from build123d import *

# Parameters (mm, degrees)
SKETCH_1_W                  = 413.2
SKETCH_1_H                  = 588.12
EXTRUDE_1_DEPTH             = 1.2
CUT_EXTRUDE_1_DEPTH         = 360.383198828
CUT_EXTRUDE_1_DEPTH_BACK    = 360.383198828
EXTRUDE_3_DEPTH             = 413.2
CUT_EXTRUDE_2_REACH         = 407.539
SKETCH_5_W                  = 413.2
SKETCH_5_H                  = 1
HOLE_WIZARD_M5_1_AT_2_COUNT = 2
HOLE_WIZARD_M5_1_AT_2_PITCH = 250
HOLE_WIZARD_M5_1_AT_3_COUNT = 2
HOLE_WIZARD_M5_1_AT_3_PITCH = 436.48692993
HOLE_WIZARD_M5_1_AT_4_COUNT = 2
HOLE_WIZARD_M5_1_AT_4_PITCH = 357.8
CUT_EXTRUDE_3_REACH         = 553.095
SKETCH_10_W                 = 80
SKETCH_10_H                 = 49
CUT_EXTRUDE_4_REACH         = 665.873
SKETCH_11_W                 = 20
SKETCH_11_H                 = 60
CUT_EXTRUDE_5_DEPTH         = 20


with BuildPart() as part:
    # 스케치1 → 보스-돌출1 (new body)
    with BuildSketch(Plane(origin=(0, 0, 0), x_dir=(1, 0, 0), z_dir=(0, 1, 0))):
        Rectangle(SKETCH_1_W, SKETCH_1_H)
    extrude(amount=EXTRUDE_1_DEPTH)

    # 스케치2 → 컷-돌출1 (cut, two sides: drawn at the far end of the back side and taken through both)
    with BuildSketch(Plane(origin=(0, 0, 0), x_dir=(0, 0, -1), z_dir=(1, 0, 0)).offset(-CUT_EXTRUDE_1_DEPTH_BACK)):
        Polygon((-293.957235481, 0), (-293.673125179, 1.2), (-294.06, 1.2), (-294.06, 0), align=None)
    extrude(amount=CUT_EXTRUDE_1_DEPTH + CUT_EXTRUDE_1_DEPTH_BACK, mode=Mode.SUBTRACT)

    # 스케치4 → 보스-돌출3 (add)
    with BuildSketch(Plane(origin=(206.6, 0, 0), x_dir=(0, 0, -1), z_dir=(1, 0, 0))):
        with BuildLine():
            Line((-293.957235481, 0), (-314.720041398, -87.696105733))
            ThreePointArc((-314.720041398, -87.696105733), (-312.832491208, -96.20326758), (-304.989056289, -100))
            Line((-304.989056289, -100), (-195.633093997, -100))
            Line((-195.633093997, -100), (-195.633093997, -149))
            Line((-195.633093997, -149), (-194.433093997, -149))
            Line((-194.433093997, -149), (-194.433093997, -98.8))
            Line((-194.433093997, -98.8), (-304.989056289, -98.8))
            ThreePointArc((-304.989056289, -98.8), (-311.891279018, -95.45887547), (-313.552323185, -87.972573045))
            Line((-313.552323185, -87.972573045), (-292.789517268, -0.276467312))
            Line((-292.789517268, -0.276467312), (-292.724061259, 0))
            Line((-292.724061259, 0), (-293.957235481, 0))
        make_face()
    extrude(amount=-EXTRUDE_3_DEPTH)

    # 스케치5 → 컷-돌출2 (cut, up to next)
    with BuildSketch(Plane(origin=(0, 1.2, 0), x_dir=(1, 0, 0), z_dir=(0, 1, 0)), mode=Mode.PRIVATE) as cut_extrude_2_sk1:
        with Locations((0, 293.56)):
            Rectangle(SKETCH_5_W, SKETCH_5_H)
    cut_extrude_2_tool1 = extrude(cut_extrude_2_sk1.sketch, amount=-CUT_EXTRUDE_2_REACH, mode=Mode.PRIVATE) & part.part
    add(cut_extrude_2_tool1.solids().sort_by_distance((0, 1.2, -293.56))[0], mode=Mode.SUBTRACT)

    # 스케치8 → M5 접시 머리 나사용 카운터싱크1 (revolve, cut)
    with BuildSketch(Plane(origin=(-125, 1.2, -213.06), x_dir=(0, 0, 1), z_dir=(1, 0, 0))):
        Polygon((0, 0), (0, 1.2), (2.75, 1.2), (2.75, 2.75), (5.2, 0.3), (5.2, 0), align=None)
    hole_wizard_m5_1 = revolve(axis=Axis((-125, 7.55, -213.06), (0, -1, 0)), mode=Mode.SUBTRACT)

    # M5 접시 머리 나사용 카운터싱크1 at 2: M5 접시 머리 나사용 카운터싱크1 ×2
    with Locations(*[(i * HOLE_WIZARD_M5_1_AT_2_PITCH, 0, 0) for i in range(1, HOLE_WIZARD_M5_1_AT_2_COUNT)]):
        add(hole_wizard_m5_1, mode=Mode.SUBTRACT)

    # M5 접시 머리 나사용 카운터싱크1 at 3: M5 접시 머리 나사용 카운터싱크1 ×2
    with Locations(*[Vector(0.5727548360724275, 0, 0.8197267213868575) * (i * HOLE_WIZARD_M5_1_AT_3_PITCH) for i in range(1, HOLE_WIZARD_M5_1_AT_3_COUNT)]):
        add(hole_wizard_m5_1, mode=Mode.SUBTRACT)

    # M5 접시 머리 나사용 카운터싱크1 at 4: M5 접시 머리 나사용 카운터싱크1 ×2
    with Locations(*[(0, 0, i * HOLE_WIZARD_M5_1_AT_4_PITCH) for i in range(1, HOLE_WIZARD_M5_1_AT_4_COUNT)]):
        add(hole_wizard_m5_1, mode=Mode.SUBTRACT)

    # 스케치10 → 컷-돌출3 (cut, up to next)
    with BuildSketch(Plane.XY.offset(195.633093997), mode=Mode.PRIVATE) as cut_extrude_3_sk1:
        with Locations((0, -124.5)):
            Rectangle(SKETCH_10_W, SKETCH_10_H)
    cut_extrude_3_tool1 = extrude(cut_extrude_3_sk1.sketch, amount=-CUT_EXTRUDE_3_REACH, mode=Mode.PRIVATE) & part.part
    add(cut_extrude_3_tool1.solids().sort_by_distance((0, -124.5, 195.633094))[0], mode=Mode.SUBTRACT)

    # 컷-돌출4: up to this plane
    cut_extrude_4_end = Plane(origin=(-206.6, -0.276467312, 292.789517268), z_dir=(0, -0.2303894266765572, -0.9730985109821345))
    # 스케치11 → 컷-돌출4 (cut, up to the surface)
    with BuildSketch(Plane.XY.offset(320), mode=Mode.PRIVATE) as cut_extrude_4_sk1:
        with Locations((-136.6, -40)):
            Rectangle(SKETCH_11_W, SKETCH_11_H)
    cut_extrude_4_tool1 = split(extrude(cut_extrude_4_sk1.sketch, amount=-CUT_EXTRUDE_4_REACH, mode=Mode.PRIVATE), bisect_by=cut_extrude_4_end, keep=Keep.BOTH, mode=Mode.PRIVATE)
    add(cut_extrude_4_tool1.solids().sort_by_distance((-136.6, -40, 320))[0], mode=Mode.SUBTRACT)
    # 스케치11 → 컷-돌출4 (cut, up to the surface)
    with BuildSketch(Plane.XY.offset(320), mode=Mode.PRIVATE) as cut_extrude_4_sk2:
        with Locations((136.6, -40)):
            Rectangle(SKETCH_11_W, SKETCH_11_H)
    cut_extrude_4_tool2 = split(extrude(cut_extrude_4_sk2.sketch, amount=-CUT_EXTRUDE_4_REACH, mode=Mode.PRIVATE), bisect_by=cut_extrude_4_end, keep=Keep.BOTH, mode=Mode.PRIVATE)
    add(cut_extrude_4_tool2.solids().sort_by_distance((136.6, -40, 320))[0], mode=Mode.SUBTRACT)

    # 스케치12 → 컷-돌출5 (cut)
    with BuildSketch(Plane(origin=(-146.6, 0, 0), x_dir=(0, 0, -1), z_dir=(1, 0, 0))):
        Polygon((-295.09164711, -10), (-296.259365323, -9.723532688), (-296.324821333, -10), (-310.530336442, -70), (-309.316935211, -70.083515414), (-309.297162219, -70), align=None)
    cut_extrude_5 = extrude(amount=CUT_EXTRUDE_5_DEPTH, mode=Mode.SUBTRACT)

    # 대칭 복사2: 컷-돌출5 across plane
    add(cut_extrude_5.mirror(Plane(origin=(0, 0, 0), x_dir=(0, 0, 1), z_dir=(1, 0, 0))), mode=Mode.SUBTRACT)


solid = part.part
Part model, mm, in its own coordinate system. Give positions to 0.01 mm unless a question says otherwise; leave off trailing zeros. Loops run counter-clockwise (first coordinate to the right, second up) from the corner with the lowest first, then second, coordinate; pieces in that order, holes last. Notation, with made-up numbers: (50.5, 33.25) -> (75.5, 33.25) arc R31 ccw to (75.5, 71.25) -> close; hole circle Ø5 at (79, -18). An arc over 180 degrees is marked (long way). Write each question's results on one line, items separated by ' | '. Start each with the question number.
Q1. Band-saw the part on B-B on x = 47.5. List the corners of the cut face in (y, z).
Q2. Pin check, flat tips, straight feed: P1, Ø24.5, axis at x = 96, y = -131.5, coming from the +Z side; P2, Ø2, axis at x = -38.5, y = -127, coming from the -Z side; P3, Ø12, axis at x = 125, z = 144.74, coming from the -Y side; P4, Ø4, axis at x = -97, y = -59.5, coming from the -Z side. Stop position of each tip, or through.
Q3. Wall check: L1, parallel to X at y = 1, z = 144; L2, parallel to Z at x = 125, y = 1; L3, parallel to X at y = 1.05, z = 144.74. Give the ranges that are in metal, low to high.
Q4. Band-saw the part on D-D on z = 77.5. List the corners of the cut face in (x, y).
Q5. Band-saw the part on A-A on y = -126. List the corners of the cut face in (x, z), plus the area to 3 significant figures.
Q6. Pull direction Y, two halves, no side cores. Call faces 1 (the face through (2.892, -96.104, 312.91)), 2 (the face through (3, -98.8, 249)), 3 (the face through (-3, 1.2, -4)), 4 (the face through (49, -124, 194.433)): +Y half, -Y half, draft (parallel to the pull), parting line (faces both ways), or undercut.
Q7. Band-saw the part on C-C on x = -28.5. List the corners of the cut face in (y, z), plus the area to 3 significant figures.
Results are:
1) outline: (-149, 194.43) -> (-98.8, 194.43) -> (-98.8, 304.99) arc R8.8 cw to (-87.97, 313.55) -> (0, 292.72) -> (0, -293.06) -> (1.2, -293.06) -> (1.2, 293.67) -> (-87.7, 314.72) arc R10 ccw to (-100, 304.99) -> (-100, 195.63) -> (-149, 195.63) -> close
2) P1: stops at z = 195.63 | P2: passes through | P3: stops at y = 0 | P4: stops at z = 306.34
3) L1: x = -206.6 to -130.15, -119.85 to 119.85, 130.15 to 206.6 | L2: z = -293.06 to -218.26, -207.86 to 139.54, 149.94 to 293.72 | L3: x = -206.6 to -130.2, -119.8 to 119.8, 130.2 to 206.6
4) outline: (-206.6, 0) -> (206.6, 0) -> (206.6, 1.2) -> (-206.6, 1.2) -> close
5) outline: (-206.6, 194.43) -> (-40, 194.43) -> (-40, 195.63) -> (-206.6, 195.63) -> close; (40, 194.43) -> (206.6, 194.43) -> (206.6, 195.63) -> (40, 195.63) -> close | area: 400 mm²
6) face 1: parting line | face 2: undercut | face 3: +Y half | face 4: draft
7) outline: (-100, 194.43) -> (-98.8, 194.43) -> (-98.8, 304.99) arc R8.8 cw to (-87.97, 313.55) -> (0, 292.72) -> (0, -293.06) -> (1.2, -293.06) -> (1.2, 293.67) -> (-87.7, 314.72) arc R10 ccw to (-100, 304.99) -> close | area: 966 mm²
